from build123d import *

# Parameters (mm, degrees)
BOSS_EXTRUDE1_DEPTH = 1
BOSS_EXTRUDE2_START = -1
SKETCH2_3_R         = 5.85
BOSS_EXTRUDE2_DEPTH = 1
SKETCH3_W           = 4
SKETCH3_H           = 1.8
BOSS_EXTRUDE3_DEPTH = 1.9
CUT_EXTRUDE1_DEPTH  = 4


with BuildPart() as part:
    # Sketch1 → Revolve1 (revolve)
    with BuildSketch(Plane.XY):
        Polygon((0, 0), (0, 5.85), (8.25, 5.85), (8.25, 5.35), (1, 5.35), (1, 4.05), (8.25, 4.05), (8.25, 3.55), (1, 3.55), (1, 2.25), (8.25, 2.25), (8.25, 1.75), (1, 1.75), (1, 0), align=None)
    revolve(axis=Axis((1, 0, 0), (-1, 0, 0)))

    # Sketch2 → Boss-Extrude1 (add)
    with BuildSketch(Plane.ZY):
        Polygon((0, 6.858921198), (-5.94, 3.429460599), (-5.94, -3.429460599), (0, -6.858921198), (5.94, -3.429460599), (5.94, 3.429460599), align=None)
    extrude(amount=BOSS_EXTRUDE1_DEPTH)

    # Sketch2<3> → Boss-Extrude2 (add)
    with BuildSketch(Plane.ZY.offset(BOSS_EXTRUDE2_START)):
        Polygon((5.94, -3.429460599), (5.94, 3.429460599), (0, 6.858921198), (-5.94, 3.429460599), (-5.94, -3.429460599), (0, -6.858921198), align=None)
        with Locations(Location((0, 0, 0), (0, 0, 90))):
            Circle(SKETCH2_3_R, mode=Mode.SUBTRACT)
    extrude(amount=BOSS_EXTRUDE2_DEPTH)

    # Sketch3 → Boss-Extrude3 (add, symmetric)
    with BuildSketch(Plane.XY):
        with Locations((-3, 0)):
            Rectangle(SKETCH3_W, SKETCH3_H)
    extrude(amount=BOSS_EXTRUDE3_DEPTH, both=True)

    # Sketch4 → Cut-Extrude1 (cut)
    with BuildSketch(Plane.ZY.offset(5)):
        with BuildLine():
            Line((-1.9, 0.9), (-1.9, 0))
            ThreePointArc((-1.9, 0), (-1.842458697, 0.464053822), (-1.673320053, 0.9))
            Line((-1.673320053, 0.9), (-1.9, 0.9))
        make_face()
        with BuildLine():
            Line((-1.9, 0), (-1.9, -0.9))
            Line((-1.9, -0.9), (-1.673320053, -0.9))
            ThreePointArc((-1.673320053, -0.9), (-1.842458697, -0.464053822), (-1.9, 0))
        make_face()
        with BuildLine():
            ThreePointArc((1.9, 0), (1.842458697, -0.464053822), (1.673320053, -0.9))
            Line((1.673320053, -0.9), (1.9, -0.9))
            Line((1.9, -0.9), (1.9, 0))
        make_face()
        with BuildLine():
            ThreePointArc((1.673320053, 0.9), (1.842458697, 0.464053822), (1.9, 0))
            Line((1.9, 0), (1.9, 0.9))
            Line((1.9, 0.9), (1.673320053, 0.9))
        make_face()
    extrude(amount=-CUT_EXTRUDE1_DEPTH, mode=Mode.SUBTRACT)


solid = part.part
The listing builds one solid part. Answer for the finished solid, in the listing's coordinates (mm). A direction names the side the tool comes from. Round coordinates to 2 decimals unless told otherwise and drop trailing zeros. Write each loop counter-clockwise with the first axis right and the second up, starting at its lowest first coordinate (ties: lowest second). Pieces come first, ordered by that corner, then holes. Notation, with made-up numbers: (69, 30.25) - (98, 30.25) arc R36 ccw to (98, 65.25) - close; hole circle Ø7 at (49, 22). An arc over 180 degrees is marked (long way). Use one line per item in the form item = value. Start each with the question number.
Item 1: A tool of negligible diameter and unlimited length cuts with its end or side. For faces 5 (the flat face through (0.014, 5.168, -2.928)), 6 (the flat face through (1, -6, 0)), from which of +Z, -Z, +X, -X, +Y, -Y can it reach the whole face along a straight path? Write none if from no direction.
Item 2: Find the intervals of material crossed by line 1 (Y direction, x = 6.75, z = 0); line 2 (X direction, y = -1, z = 0.75), in increasing order. Write a range as [from, to].
Item 3: A cutting plane is placed at A-A (x = 2.5). Write down the section's boundary in (y, z), plus the area to 3 significant figures.
Item 4: A cutting plane is placed at D-D (y = -2.5). Write down the section's boundary in (x, z), plus the area to 3 significant figures.
Item 5: Flat-ended cylindrical pins translate along their axes: pin 1 Ø1.8 at (y, z) = (-0.5, 0.5) entering from +X; pin 2 Ø5.5 at (y, z) = (1.5, -2) entering from +X; pin 3 Ø2.5 at (x, z) = (-3.5, 0.5) entering from -Y; pin 4 Ø1.5 at (y, z) = (3, -4) entering from -X. Find the tip coordinate at first contact, or state that the pin passes through.
Item 6: Determine the mould class of faces 1 (the flat face through (-3, -0.9, 0)), 2 (the flat face through (0.01, 5.12, 3.01)), 3 (the flat face through (1, 2, -4)), 4 (the flat face through (-1, -1.4, -0.1)) for opening direction Y: +Y half, -Y half, draft (parallel to the pull), parting line (faces both ways), or undercut.
Item 7: A cutting plane is placed at B-B (x = -1.5). Write down the section's boundary in (y, z), plus the area to 3 significant figures.
Item 8: A cutting plane is placed at C-C (z = -4.75). Write down the section's boundary in (x, y).
The answers:
q1.face_5 = -Z, +X, -X, +Y
q1.face_6 = +X
q2.line_1 = [-5.85, -5.35], [-4.05, -3.55], [-2.25, -1.75], [1.75, 2.25], [3.55, 4.05], [5.35, 5.85]
q2.line_2 = [-1, 1]
q3.outline = circle Ø11.7 at (0, 0); circle Ø8.1 at (0, 0); circle Ø4.5 at (0, 0); hole circle Ø10.7 at (0, 0); hole circle Ø7.1 at (0, 0); hole circle Ø3.5 at (0, 0)
q3.area = 35.8 mm^2
q4.outline = (-1, -5.94) - (1, -5.94) - (1, -5.29) - (8.25, -5.29) - (8.25, -4.73) - (1, -4.73) - (1, -3.19) - (8.25, -3.19) - (8.25, -2.52) - (1, -2.52) - (1, 2.52) - (8.25, 2.52) - (8.25, 3.19) - (1, 3.19) - (1, 4.73) - (8.25, 4.73) - (8.25, 5.29) - (1, 5.29) - (1, 5.94) - (-1, 5.94) - close
q4.area = 41.5 mm^2
q5.pin_1 = 1
q5.pin_2 = 8.25
q5.pin_3 = -0.9
q5.pin_4 = -1
q6.face_1 = -Y half
q6.face_2 = +Y half
q6.face_3 = undercut
q6.face_4 = draft
q7.outline = (-0.9, -1.67) arc R1.9 ccw to (0.9, -1.67) - (0.9, 1.67) arc R1.9 ccw to (-0.9, 1.67) - close
q7.area = 6.57 mm^2
q8.outline = (-1, -4.12) - (1, -4.12) - (1, -3.41) - (8.25, -3.41) - (8.25, -2.46) - (1, -2.46) - (1, 2.46) - (8.25, 2.46) - (8.25, 3.41) - (1, 3.41) - (1, 4.12) - (-1, 4.12) - close
